Study the drawing (mm; zero at the part's minimum x, y, z) and answer. A direction names the side the tool comes from. Round coordinates to 2 decimals unless told otherwise and drop trailing zeros. Loops run counter-clockwise (first coordinate to the right, second up) from the corner with the lowest first, then second, coordinate; pieces in that order, holes last. Notation, with made-up numbers: (4.25, -18) -> (26.25, -18) arc R21 cw to (26.25, -4) -> close; hole circle Ø6 at (-40, 60.5). An arc over 180 degrees is marked (long way). Write each question's results on one line, items separated by ' | '. Start each with the question number.
(1) Determine the mould class of the marked faces 1, 2, 3 and 4 for opening direction Y: released by +Y, released by -Y, zero draft, split by the parting line, or undercut.
(2) Straight lines are drawn through the part: probe 1 along X at (y, z) = (42, 6.5); probe 2 along X at (y, z) = (11.43, 0.7). For each, find the intervals that lie inside material, in ascending order.
(3) The part is cut by section B-B (y = 22). Determine the outline of the cut face in (x, z).
(4) For the marked faces 5 and 6, determine the directions among +Z, -Z, +X, -X, +Y, -Y from which every point of the face is accessible in a straight line to the end or side of a thin tool.
(5) The part is cut by section A-A (z = 4.5). Determine the outline of the cut face in (x, y).
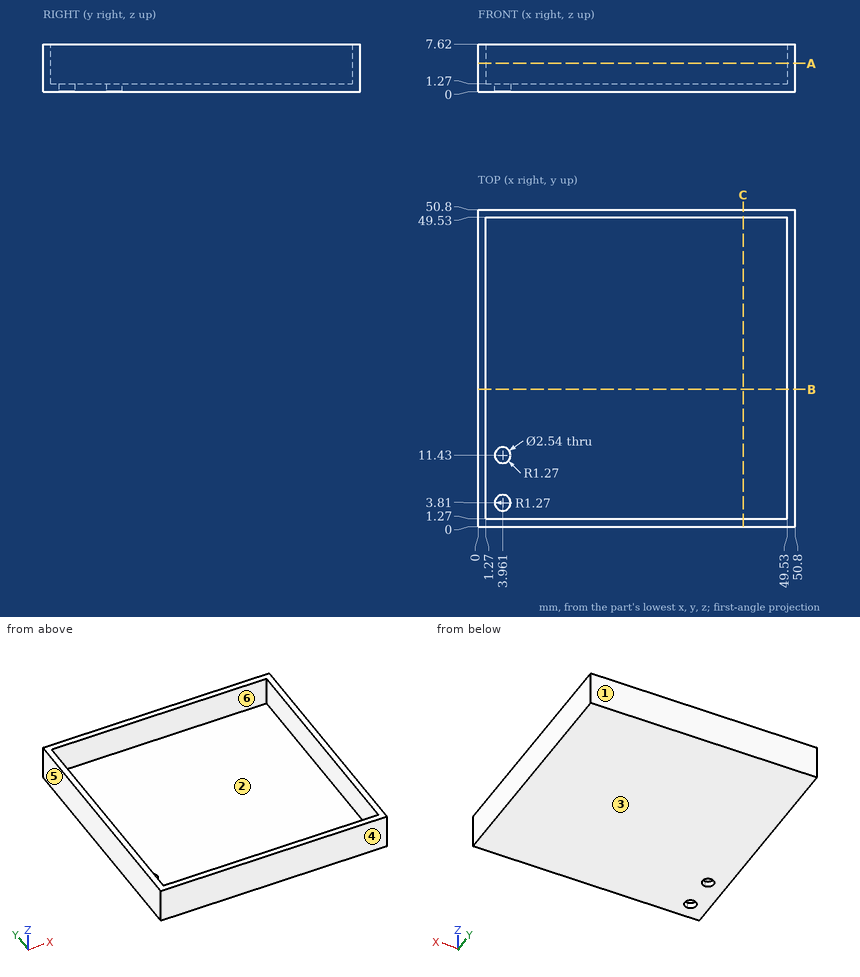
Checked values:
1) face 1: released by +Y | face 2: undercut | face 3: zero draft | face 4: released by -Y
2) probe 1: x = 0 to 1.27, 49.53 to 50.8 | probe 2: x = 0 to 2.69, 5.23 to 50.8
3) outline: (0, 0) -> (50.8, 0) -> (50.8, 7.62) -> (49.53, 7.62) -> (49.53, 1.27) -> (1.27, 1.27) -> (1.27, 7.62) -> (0, 7.62) -> close
4) face 5: +Z, -Z, -X, +Y, -Y | face 6: +Z
5) outline: (0, 0) -> (50.8, 0) -> (50.8, 50.8) -> (0, 50.8) -> close; hole (1.27, 1.27) -> (49.53, 1.27) -> (49.53, 49.53) -> (1.27, 49.53) -> close
